```python
from build123d import *

# Parameters (mm, degrees)
SKETCH1_W           = 50.8
SKETCH1_H           = 25.4
SKETCH1_W_2         = 45.72
SKETCH1_H_2         = 20.32
EXTRUDE_THIN1_DEPTH = 53.975
CUT_EXTRUDE1_DEPTH  = 26.4
SKETCH3_W           = 50.8
SKETCH3_H           = 50.8
CUT_EXTRUDE2_DEPTH  = 26.4
SKETCH5_R           = 2.4765
CUT_EXTRUDE4_DEPTH  = 26.4


with BuildPart() as part:
    # Sketch1 → Extrude-Thin1 (new body, symmetric)
    with BuildSketch(Plane(origin=(0, 0, 0), x_dir=(1, 0, 0), z_dir=(0, 1, 0))):
        Rectangle(SKETCH1_W, SKETCH1_H)
        Rectangle(SKETCH1_W_2, SKETCH1_H_2, mode=Mode.SUBTRACT)
    extrude(amount=EXTRUDE_THIN1_DEPTH, both=True)

    # Sketch2 → Cut-Extrude1 (cut, through all)
    with BuildSketch(Plane.XY.offset(12.7)):
        Polygon((-25.4, 53.975), (25.4, 53.975), (-25.4, 40.363181024), align=None)
    extrude(amount=-CUT_EXTRUDE1_DEPTH, mode=Mode.SUBTRACT)

    # Sketch3 → Cut-Extrude2 (cut, through all)
    with BuildSketch(Plane.XY.offset(12.7)):
        with Locations((0, -28.575)):
            Rectangle(SKETCH3_W, SKETCH3_H)
    extrude(amount=-CUT_EXTRUDE2_DEPTH, mode=Mode.SUBTRACT)

    # Sketch5 → Cut-Extrude4 (cut, through all)
    with BuildSketch(Plane(origin=(0, 0, -12.7), x_dir=(-1, 0, 0), z_dir=(0, 0, -1))):
        with Locations((0, 9.525)):
            Circle(SKETCH5_R)
        with Locations((0, 34.021083021)):
            Circle(SKETCH5_R)
    extrude(amount=-CUT_EXTRUDE4_DEPTH, mode=Mode.SUBTRACT)


solid = part.part
```
Verification items for the finished model (mm, model axes). A direction names the side the tool comes from. Round coordinates to 2 decimals unless told otherwise and drop trailing zeros. Write each loop counter-clockwise with the first axis right and the second up, starting at its lowest first coordinate (ties: lowest second). Pieces come first, ordered by that corner, then holes. Notation, with made-up numbers: (23, -35.5) -> (71, -35.5) arc R23 ccw to (71, -23.5) -> close; hole circle Ø4 at (81, -22.5). An arc over 180 degrees is marked (long way). Write each question's results on one line, items separated by ' | '. Start each with the question number.
1. Set-up check for faces 1 (the flat face through (0, 19, -12.7)), 2 (the flat face through (22.86, 25, 0)): record each of +Z, -Z, +X, -X, +Y, -Y from which the full face is reachable in a straight line by a thin tool's end or side.
2. Cross-section at B-B (x = 0). Enter the section's corners in (y, z) (1 decimal).
3. Cross-section at C-C (y = 2.5). Enter the section's corners in (x, z), then the cut area to 3 significant figures.
4. Cross-section at D-D (x = 20). Enter the section's corners in (y, z) (3 decimals).
5. Draft check along X on faces 3 (the cylindrical face through (0.322, 36.477, -11.448)), 4 (the flat face through (-25.4, 19, 0)), 5 (the flat face through (25.4, 26, 0)), 6 (the flat face through (-0.1, -3.175, 10.4)). Enter one of: +X half, -X half, draft (parallel to the pull), parting line (faces both ways), or undercut.
6. Cross-section at A-A (z = 7.75). Enter the section's corners in (x, y) (3 decimals), then the cut area to 3 significant figures.
7. Material ranges on probe 1 along X at (y, z) = (31, 7); probe 2 along Z at (x, y) = (9, 44.5); probe 3 along Y at (x, z) = (0, 10.7) (1 decimal), recorded low to high. Write a range as from..to.
8. Depth check by flat-ended pin: P1, Ø12, axis at x = 11, z = 8.5, coming from the +Y side. Enter the tip coordinate at first touch or a pass-through.
Solutions:
1) face 1: -Z, +X, -X, +Y, -Y | face 2: +Y, -Y
2) outline: (-3.2, -12.7) -> (7, -12.7) -> (7, -10.2) -> (-3.2, -10.2) -> close; (-3.2, 10.2) -> (7, 10.2) -> (7, 12.7) -> (-3.2, 12.7) -> close; (12, -12.7) -> (31.5, -12.7) -> (31.5, -10.2) -> (12, -10.2) -> close; (12, 10.2) -> (31.5, 10.2) -> (31.5, 12.7) -> (12, 12.7) -> close; (36.5, -12.7) -> (47.2, -12.7) -> (47.2, -10.2) -> (36.5, -10.2) -> close; (36.5, 10.2) -> (47.2, 10.2) -> (47.2, 12.7) -> (36.5, 12.7) -> close
3) outline: (-25.4, -12.7) -> (25.4, -12.7) -> (25.4, 12.7) -> (-25.4, 12.7) -> close; hole (-22.86, -10.16) -> (22.86, -10.16) -> (22.86, 10.16) -> (-22.86, 10.16) -> close | area: 361 mm2
4) outline: (-3.175, -12.7) -> (52.528, -12.7) -> (52.528, -10.16) -> (-3.175, -10.16) -> close; (-3.175, 10.16) -> (52.528, 10.16) -> (52.528, 12.7) -> (-3.175, 12.7) -> close
5) face 3: undercut | face 4: -X half | face 5: +X half | face 6: draft
6) outline: (-25.4, -3.175) -> (-22.86, -3.175) -> (-22.86, 41.044) -> (-25.4, 40.363) -> close; (22.86, -3.175) -> (25.4, -3.175) -> (25.4, 53.975) -> (22.86, 53.294) -> close | area: 256 mm2
7) probe 1: x = -25.4..-22.86, 22.86..25.4 | probe 2: z = -12.7..-10.16, 10.16..12.7 | probe 3: y = -3.2..7, 12..31.5, 36.5..47.2
8) P1: stops at y = 51.66
